```python
from build123d import *

# Parameters (mm, degrees)
SKETCH1_W           = 25.4
SKETCH1_H           = 50.8
SKETCH1_W_2         = 19.05
SKETCH1_H_2         = 44.45
BOSS_EXTRUDE1_DEPTH = 508
SKETCH3_R           = 3.175
CUT_EXTRUDE1_DEPTH  = 512.165139656
SKETCH4_R           = 2.4638
CUT_EXTRUDE2_DEPTH  = 512.165139656
CUT_EXTRUDE3_DEPTH  = 512.165139656
LPATTERN1_COUNT     = 6
LPATTERN1_PITCH     = 59.69
SKETCH6_R           = 2.5796875
CUT_EXTRUDE4_DEPTH  = 512.165139656


with BuildPart() as part:
    # Sketch1 → Boss-Extrude1 (new body)
    with BuildSketch(Plane(origin=(0, 0, 0), x_dir=(1, 0, 0), z_dir=(0, 1, 0))):
        with Locations((12.7, 25.4)):
            Rectangle(SKETCH1_W, SKETCH1_H)
        with Locations((12.7, 25.4)):
            Rectangle(SKETCH1_W_2, SKETCH1_H_2, mode=Mode.SUBTRACT)
    extrude(amount=BOSS_EXTRUDE1_DEPTH)

    # Sketch3 → Cut-Extrude1 (cut, through all)
    with BuildSketch(Plane.XY):
        with Locations((12.7, 177.8)):
            Circle(SKETCH3_R)
        with Locations((12.7, 12.7)):
            Circle(SKETCH3_R)
    extrude(amount=-CUT_EXTRUDE1_DEPTH, mode=Mode.SUBTRACT)

    # Sketch4 → Cut-Extrude2 (cut, through all)
    with BuildSketch(Plane.ZY):
        with Locations((-25.4, 457.2)):
            Circle(SKETCH4_R)
        with Locations((-25.4, 495.3)):
            Circle(SKETCH4_R)
    extrude(amount=-CUT_EXTRUDE2_DEPTH, mode=Mode.SUBTRACT)

    # Sketch5 → Cut-Extrude3 (cut, through all)
    with BuildSketch(Plane(origin=(25.4, 0, 0), x_dir=(0, 0, -1), z_dir=(1, 0, 0))):
        Polygon((41.91, 88.928211777), (8.89, 69.864105889), (41.91, 50.8), align=None)
        Polygon((41.91, 99.193499563), (8.89, 118.257605452), (8.89, 80.129393675), align=None)
    cut_extrude3 = extrude(amount=-CUT_EXTRUDE3_DEPTH, mode=Mode.SUBTRACT)

    # LPattern1: Cut-Extrude3 ×6
    with Locations(*[(0, i * LPATTERN1_PITCH, 0) for i in range(1, LPATTERN1_COUNT)]):
        add(cut_extrude3, mode=Mode.SUBTRACT)

    # Sketch6 → Cut-Extrude4 (cut, through all)
    with BuildSketch(Plane(origin=(0, 0, -50.8), x_dir=(-1, 0, 0), z_dir=(0, 0, -1))):
        with Locations((-12.7, 431.8)):
            Circle(SKETCH6_R)
        with Locations((-12.7, 338.053316528)):
            Circle(SKETCH6_R)
    extrude(amount=-CUT_EXTRUDE4_DEPTH, mode=Mode.SUBTRACT)


solid = part.part
```
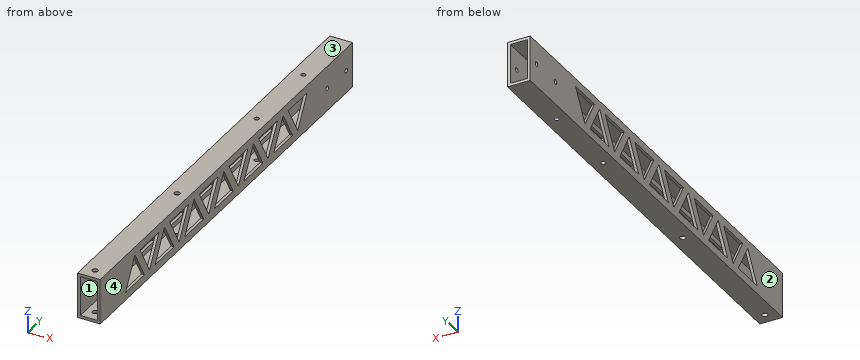
Geometry: final body of the model. Coordinates: model frame, mm. Face numbers are marked on the shaded views. Coordinates: 2 decimals unless noted, no trailing zeros. Order: outer loops, then holes, each group sorted by start corner. A loop starts at its lowest first (then second) coordinate and runs counter-clockwise, first axis right, second up. Notation, with made-up numbers: M -30.5,-34 L 25.5,-34 A11 ccw 25.5,-21 Z; hole C 0,-31.5 d10. An arc over 180 degrees is marked long. Answer in a Markdown table with one row per item. Add a question column.
Q1. Section query B-B on y = 204. Return the cut outline in (x, z) (3 decimals).
Q2. Section query A-A on y = 408. Return the cut outline in (x, z) (3 decimals).
Q3. Line query: L1, parallel to Y at x = 12.7, z = -48.25 (3 decimals); L2, parallel to Z at x = 11, y = 163.5 (3 decimals); L3, parallel to X at y = 431.8, z = -1.7. Output: solid intervals per line, ascending.
Q4. Mould query, pull axis X, two halves, no side actions, for the marked faces 1, 2, 3 and 4. Classes: released by +X, released by -X, zero draft, split by the parting line, or undercut.
Q5. Section query C-C on z = -16. Count the separate pieces of the cut face and the enclosed holes in it, and give its area (3 significant figures).
Q6. Contact query for a flat-ended pin moving along its axis: P1, Ø6.5, axis at y = 495.3, z = -25.4, coming from the -X side. Output: stop coordinate, or through.
Completed:
| question | item | result |
|---|---|---|
| 1 | outline | M 0,-50.8 L 25.4,-50.8 L 25.4,-41.91 L 22.225,-41.91 L 22.225,-47.625 L 3.175,-47.625 L 3.175,-41.91 L 0,-41.91 Z; M 0,-34.448 L 3.175,-34.448 L 3.175,-16.668 L 0,-16.668 Z; M 0,-8.89 L 3.175,-8.89 L 3.175,-3.175 L 22.225,-3.175 L 22.225,-8.89 L 25.4,-8.89 L 25.4,0 L 0,0 Z; M 22.225,-34.448 L 25.4,-34.448 L 25.4,-16.668 L 22.225,-16.668 Z |
| 2 | outline | M 0,-50.8 L 25.4,-50.8 L 25.4,-23.972 L 22.225,-23.972 L 22.225,-47.625 L 3.175,-47.625 L 3.175,-23.972 L 0,-23.972 Z; M 0,-8.89 L 3.175,-8.89 L 3.175,-3.175 L 22.225,-3.175 L 22.225,-8.89 L 25.4,-8.89 L 25.4,0 L 0,0 Z |
| 3 | L1 | y = 0 to 9.525, 15.875 to 174.625, 180.975 to 335.474, 340.633 to 429.22, 434.38 to 508 |
| 3 | L2 | z = -50.8 to -47.625, -3.175 to 0 |
| 3 | L3 | x = 0 to 10.12, 15.28 to 25.4 |
| 4 | face 1 | undercut |
| 4 | face 2 | released by -X |
| 4 | face 3 | zero draft |
| 4 | face 4 | released by +X |
| 5 | separate pieces | 26 |
| 5 | enclosed holes | 0 |
| 5 | area | 1,770 mm2 |
| 6 | P1 | stops at x = 0 |
